```python
from build123d import *

# Parameters (mm, degrees)
F0_W     = 101.6
F0_H     = 101.6
F1_DEPTH = 44.45
F3_D     = 12.7
F4_W     = 50.8
F4_H     = 50.8
F5_DEPTH = 88.9
F7_D     = 6.35


with BuildPart() as f1:
    # F0 (on Front) → F1 (new body)
    with BuildSketch(Plane.XZ):
        Rectangle(F0_W, F0_H)
    extrude(amount=F1_DEPTH)

    # F3 (through all)
    with Locations(Plane.XZ.offset(44.45)):
        with Locations((0, 0)):
            Hole(F3_D / 2)

    # F4 (on face) → F5 (cut)
    with BuildSketch(Plane.XZ.offset(44.45)):
        with Locations((25.4, 25.4)):
            Rectangle(F4_W, F4_H)
    extrude(amount=-F5_DEPTH, mode=Mode.SUBTRACT)

    # F7 (through all)
    with Locations(Plane.XZ.offset(44.45)):
        with Locations((-25.4, -25.4)):
            Hole(F7_D / 2)


solid = f1.part
```
Input: part model. Units: mm. Frame: model coordinates. A direction names the side the tool comes from. Coordinates: 2 decimals unless noted, no trailing zeros. Write each loop counter-clockwise with the first axis right and the second up, starting at its lowest first coordinate (ties: lowest second). Pieces come first, ordered by that corner, then holes. Notation, with made-up numbers: M -0.5,87.25 L 40.5,87.25 A10 cw 40.5,102.25 Z; hole C 46,-28 d1. An arc over 180 degrees is marked long. Use one line per item in the form item = value.
Q1. First-contact query: pin 1 (10 mm diameter, centred on x = 26, y = -21.5, fed in from +Z); pin 2 (22 mm diameter, centred on y = -27.5, z = 23, fed in from +X). Flat tips, straight axial feed; report the tip coordinate or a pass-through.
Answer below:
pin_1 = 0
pin_2 = 0
Q2. Material intervals for probe 1 along Z at (x, y) = (-25.4, -26.5) (3 decimals); probe 2 along X at (y, z) = (-34, -25); probe 3 along Z at (x, y) = (40.5, -16.5), sorted ascending. Write a range as from..to.
Answer below:
probe_1 = -50.8..-28.575, -22.225..50.8
probe_2 = -50.8..-28.55, -22.25..50.8
probe_3 = -50.8..0
Q3. Draft query along Z for faces 1 (the face through (-4.34, -21.914, -4.636)), 2 (the face through (-1, -22, -50.8)), 3 (the face through (-12, -44.45, -11)). Return one class per face: released by +Z, released by -Z, zero draft, split by the parting line, or undercut.
Answer below:
face_1 = undercut
face_2 = released by -Z
face_3 = zero draft
Q4. Section D-D (x = 29). Return loops of the section in (y, z), plus the area to 3 significant figures.
Answer below:
outline = M -44.45,-50.8 L 0,-50.8 L 0,0 L -44.45,0 Z
area = 2,260 mm²
Q5. Set-up query: faces 4 (the face through (50.8, -22, -26)), 5 (the face through (28, -23, 0)). Return all of +Z, -Z, +X, -X, +Y, -Y with unobstructed straight access to the full face (end or side cutting, diameter ignored); none if empty.
Answer below:
face_4 = +Z, -Z, +X, +Y, -Y
face_5 = +Z, +X, +Y, -Y
Q6. Section C-C (z = 24.5). Return loops of the section in (x, y).
Answer below:
outline = M -50.8,-44.45 L 0,-44.45 L 0,0 L -50.8,0 Z
Q7. Section A-A (z = -25.4). Return loops of the section in (x, y) (3 decimals).
Answer below:
outline = M -50.8,-44.45 L -28.575,-44.45 L -28.575,0 L -50.8,0 Z; M -22.225,-44.45 L 50.8,-44.45 L 50.8,0 L -22.225,0 Z
Q8. Section B-B (y = -22). Return loops of the section in (x, z) (3 decimals).
Answer below:
outline = M -50.8,-50.8 L 50.8,-50.8 L 50.8,0 L 6.35,0 A6.35 cw long 0,6.35 L 0,50.8 L -50.8,50.8 Z; hole C -25.4,-25.4 d6.35
